The model under review builds one solid part; all positions refer to its coordinate system, in mm. Face numbers are marked on the shaded views. A direction names the side the tool comes from. Round coordinates to 2 decimals unless told otherwise and drop trailing zeros. Write each loop counter-clockwise with the first axis right and the second up, starting at its lowest first coordinate (ties: lowest second). Pieces come first, ordered by that corner, then holes. Notation, with made-up numbers: M 51.25,71 L 106.25,71 A8 cw 106.25,83 Z; hole C -13.75,13.25 d9. An arc over 180 degrees is marked long. Write item = value, one per line. Start each with the question number.
Item 1: To check wall thickness, follow line 1 along X through (y, z) = (-15.75, -0.1); line 2 along Y through (x, z) = (43.75, -0.25); line 3 along Y through (x, z) = (-14, 3). State the ranges of each line that lie inside material, in increasing order.
Item 2: Tool access review of the marked faces 1 and 2: name each direction out of +Z, -Z, +X, -X, +Y, -Y from which nothing blocks a thin tool from reaching the whole face with its end or side.
Item 3: Take a section at A-A, the plane z = -5.75. Give the boundary of the cut face in (x, y), plus the area to 3 significant figures.
Item 4: Take a section at C-C, the plane z = 6.5. Give the number of separate pieces and of enclosed holes in the cut face, plus the area to 3 significant figures.
Item 5: The part is to be moulded in two halves that separate along Y. For the marked faces 3, 4 and 5, say which applies: +Y half, -Y half, draft (parallel to the pull), parting line (faces both ways), or undercut.
Item 6: For pin 1 Ø2 at (x, y) = (43.5, -16.5) entering from -Z; pin 2 Ø3.5 at (x, z) = (45, -3) entering from -Y; pin 3 Ø16 at (x, y) = (-20, 2.5) entering from +Z, all flat-tipped, find the tip position at first contact; note any pin that passes through.
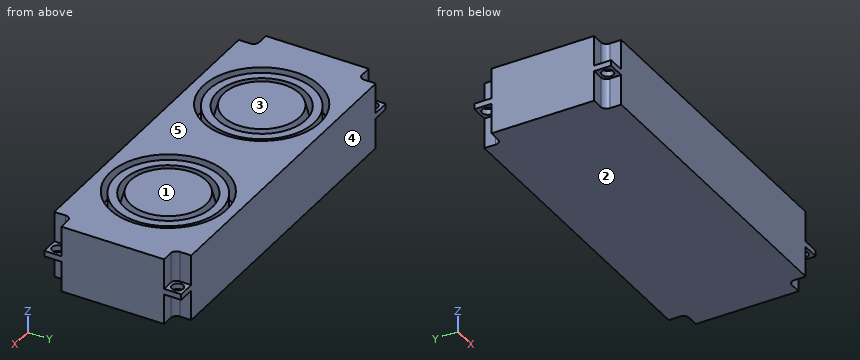
from build123d import *

# Parameters (mm, degrees)
SKETCH1_W               = 92
SKETCH1_H               = 36
BOSS_EXTRUDE1_DEPTH     = 8.75
CUT_EXTRUDE1_DEPTH      = 53.404675364
CUT_EXTRUDE1_DEPTH_BACK = 53.404675364
SKETCH2_R               = 1.5
SKETCH3_R               = 1.5
CUT_EXTRUDE2_DEPTH      = 8
CUT_EXTRUDE3_START      = -8
SKETCH4_R               = 1.5
CUT_EXTRUDE3_DEPTH      = 8
SKETCH5_R               = 15.355410725
CUT_EXTRUDE4_DEPTH      = 6.5
SKETCH6_R               = 13.829083231
SKETCH6_R_2             = 11.607285571
BOSS_EXTRUDE2_DEPTH     = 6
SKETCH7_R               = 11.607285571
BOSS_EXTRUDE3_DEPTH     = 6.2
BOSS_EXTRUDE3_TAPER     = 15


with BuildPart() as part:
    # Sketch1 → Boss-Extrude1 (new, symmetric)
    with BuildSketch(Plane.XY):
        Rectangle(SKETCH1_W, SKETCH1_H)
    extrude(amount=BOSS_EXTRUDE1_DEPTH, both=True)

    # Sketch2 → Cut-Extrude1 (cut, two sides: drawn at the far end of the back side and taken through both)
    with BuildSketch(Plane.XY.offset(8.75).offset(-CUT_EXTRUDE1_DEPTH_BACK)):
        with Locations((43.75, 15.75)):
            Circle(SKETCH2_R)
        with Locations((43.75, -15.75)):
            Circle(SKETCH2_R)
        with Locations((-43.75, -15.75)):
            Circle(SKETCH2_R)
        with Locations((-43.75, 15.75)):
            Circle(SKETCH2_R)
    extrude(amount=CUT_EXTRUDE1_DEPTH + CUT_EXTRUDE1_DEPTH_BACK, mode=Mode.SUBTRACT)

    # Sketch3 → Cut-Extrude2 (cut)
    # profile 1 of 4: a face of its own
    with BuildSketch(Plane.XY.offset(8.75)):
        with BuildLine():
            Line((-41.5, 18), (-46, 18))
            Line((-46, 18), (-46, 13.5))
            Line((-46, 13.5), (-43, 13.5))
            ThreePointArc((-43, 13.5), (-41.939339828, 13.939339828), (-41.5, 15))
            Line((-41.5, 15), (-41.5, 18))
        make_face()
        with Locations((-43.75, 15.75)):
            Circle(SKETCH3_R, mode=Mode.SUBTRACT)
    # profile 2 of 4: a face of its own
    with BuildSketch(Plane.XY.offset(8.75)):
        with BuildLine():
            Line((41.5, 18), (41.5, 15))
            ThreePointArc((41.5, 15), (41.939339828, 13.939339828), (43, 13.5))
            Line((43, 13.5), (46, 13.5))
            Line((46, 13.5), (46, 18))
            Line((46, 18), (41.5, 18))
        make_face()
        with Locations((43.75, 15.75)):
            Circle(SKETCH3_R, mode=Mode.SUBTRACT)
    # profile 3 of 4: a face of its own
    with BuildSketch(Plane.XY.offset(8.75)):
        with BuildLine():
            Line((-41.5, -18), (-41.5, -15))
            ThreePointArc((-41.5, -15), (-41.939339828, -13.939339828), (-43, -13.5))
            Line((-43, -13.5), (-46, -13.5))
            Line((-46, -13.5), (-46, -18))
            Line((-46, -18), (-41.5, -18))
        make_face()
        with Locations((-43.75, -15.75)):
            Circle(SKETCH3_R, mode=Mode.SUBTRACT)
    # profile 4 of 4: a face of its own
    with BuildSketch(Plane.XY.offset(8.75)):
        with BuildLine():
            Line((41.5, -18), (46, -18))
            Line((46, -18), (46, -13.5))
            Line((46, -13.5), (43, -13.5))
            ThreePointArc((43, -13.5), (41.939339828, -13.939339828), (41.5, -15))
            Line((41.5, -15), (41.5, -18))
        make_face()
        with Locations((43.75, -15.75)):
            Circle(SKETCH3_R, mode=Mode.SUBTRACT)
    extrude(amount=-CUT_EXTRUDE2_DEPTH, mode=Mode.SUBTRACT)

    # Sketch4 → Cut-Extrude3 (cut)
    # profile 1 of 4: a face of its own
    with BuildSketch(Plane(origin=(0, 0, -8.75), x_dir=(-1, 0, 0), z_dir=(0, 0, -1)).offset(CUT_EXTRUDE3_START)):
        with BuildLine():
            Line((46, 18), (41.5, 18))
            Line((41.5, 18), (41.5, 15))
            ThreePointArc((41.5, 15), (41.939339828, 13.939339828), (43, 13.5))
            Line((43, 13.5), (46, 13.5))
            Line((46, 13.5), (46, 18))
        make_face()
        with Locations(Location((43.75, 15.75, 0), (0, 0, 180))):
            Circle(SKETCH4_R, mode=Mode.SUBTRACT)
    # profile 2 of 4: a face of its own
    with BuildSketch(Plane(origin=(0, 0, -8.75), x_dir=(-1, 0, 0), z_dir=(0, 0, -1)).offset(CUT_EXTRUDE3_START)):
        with BuildLine():
            Line((-41.5, 15), (-41.5, 18))
            Line((-41.5, 18), (-46, 18))
            Line((-46, 18), (-46, 13.5))
            Line((-46, 13.5), (-43, 13.5))
            ThreePointArc((-43, 13.5), (-41.939339828, 13.939339828), (-41.5, 15))
        make_face()
        with Locations(Location((-43.75, 15.75, 0), (0, 0, 180))):
            Circle(SKETCH4_R, mode=Mode.SUBTRACT)
    # profile 3 of 4: a face of its own
    with BuildSketch(Plane(origin=(0, 0, -8.75), x_dir=(-1, 0, 0), z_dir=(0, 0, -1)).offset(CUT_EXTRUDE3_START)):
        with BuildLine():
            Line((41.5, -15), (41.5, -18))
            Line((41.5, -18), (46, -18))
            Line((46, -18), (46, -13.5))
            Line((46, -13.5), (43, -13.5))
            ThreePointArc((43, -13.5), (41.939339828, -13.939339828), (41.5, -15))
        make_face()
        with Locations(Location((43.75, -15.75, 0), (0, 0, 180))):
            Circle(SKETCH4_R, mode=Mode.SUBTRACT)
    # profile 4 of 4: a face of its own
    with BuildSketch(Plane(origin=(0, 0, -8.75), x_dir=(-1, 0, 0), z_dir=(0, 0, -1)).offset(CUT_EXTRUDE3_START)):
        with BuildLine():
            Line((-46, -18), (-41.5, -18))
            Line((-41.5, -18), (-41.5, -15))
            ThreePointArc((-41.5, -15), (-41.939339828, -13.939339828), (-43, -13.5))
            Line((-43, -13.5), (-46, -13.5))
            Line((-46, -13.5), (-46, -18))
        make_face()
        with Locations(Location((-43.75, -15.75, 0), (0, 0, 180))):
            Circle(SKETCH4_R, mode=Mode.SUBTRACT)
    extrude(amount=CUT_EXTRUDE3_DEPTH, mode=Mode.SUBTRACT)

    # Sketch5 → Cut-Extrude4 (cut)
    with BuildSketch(Plane.XY.offset(8.75)):
        with Locations((-21.003558343, 0)):
            Circle(SKETCH5_R)
        with Locations((21.003558343, 0)):
            Circle(SKETCH5_R)
    extrude(amount=-CUT_EXTRUDE4_DEPTH, mode=Mode.SUBTRACT)

    # Sketch6 → Boss-Extrude2 (add)
    with BuildSketch(Plane.XY.offset(2.25)):
        with Locations((-21.003558343, 0)):
            Circle(SKETCH6_R)
        with Locations((-21.003558343, 0)):
            Circle(SKETCH6_R_2, mode=Mode.SUBTRACT)
    boss_extrude2 = extrude(amount=BOSS_EXTRUDE2_DEPTH)

    # Sketch7 → Boss-Extrude3 (add)
    with BuildSketch(Plane.XY.offset(2.25)):
        with Locations((-21.003558343, 0)):
            Circle(SKETCH7_R)
    boss_extrude3 = extrude(amount=BOSS_EXTRUDE3_DEPTH, taper=BOSS_EXTRUDE3_TAPER)

    # Mirror2: Boss-Extrude2, Boss-Extrude3 across plane
    add(boss_extrude2.mirror(Plane(origin=(0, 0, 0), x_dir=(0, 0, 1), z_dir=(1, 0, 0))))
    add(boss_extrude3.mirror(Plane(origin=(0, 0, 0), x_dir=(0, 0, 1), z_dir=(1, 0, 0))))


solid = part.part
Response values:
q1.line_1 = -46 to -45.25, -42.25 to 42.25, 45.25 to 46
q1.line_2 = -18 to -17.25, -14.25 to 14.25, 17.25 to 18
q1.line_3 = -18 to -13.67, -11.92 to -9.26, -9 to 9, 9.26 to 11.92, 13.67 to 18
q2.face_1 = +Z
q2.face_2 = -Z, +X, -X, +Y, -Y
q3.outline = M -46,-13.5 L -43,-13.5 A1.5 cw -41.5,-15 L -41.5,-18 L 41.5,-18 L 41.5,-15 A1.5 cw 43,-13.5 L 46,-13.5 L 46,13.5 L 43,13.5 A1.5 cw 41.5,15 L 41.5,18 L -41.5,18 L -41.5,15 A1.5 cw -43,13.5 L -46,13.5 Z
q3.area = 3,230 mm2
q4.separate_pieces = 5
q4.enclosed_holes = 4
q4.area = 2,800 mm2
q5.face_3 = undercut
q5.face_4 = +Y half
q5.face_5 = draft
q6.pin_1 = -0.75
q6.pin_2 = -13.5
q6.pin_3 = 8.45
